Design review of the part built by this model. Coordinates are the model's own, in mm. A direction names the side the tool comes from. Coordinates: 2 decimals unless noted, no trailing zeros. Write each loop counter-clockwise with the first axis right and the second up, starting at its lowest first coordinate (ties: lowest second). Pieces come first, ordered by that corner, then holes. Notation, with made-up numbers: (12, 41) - (28, 41) arc R24 ccw to (28, 76) - close; hole circle Ø11 at (5, -30.5). An arc over 180 degrees is marked (long way). Use a Markdown table: item, result.
from build123d import *

# Parameters (mm, degrees)
BOSS_EXTRUDE1_DEPTH     = 20
CUT_EXTRUDE1_DEPTH      = 31.882754065
CUT_EXTRUDE1_DEPTH_BACK = 31.882754065
SKETCH2_R               = 2
SKETCH2_W               = 2
SKETCH2_H               = 5
FILLET1_R               = 2
FILLET2_R               = 0.5


with BuildPart() as part:
    # Sketch1 → Boss-Extrude1 (new body)
    with BuildSketch(Plane(origin=(0, 0, 0), x_dir=(1, 0, 0), z_dir=(0, 1, 0))):
        with BuildLine():
            Line((1.933321902, 6.18565004), (21.840134803, 7.875133355))
            ThreePointArc((21.840134803, 7.875133355), (22.103064319, 7.689578117), (21.96535024, 7.398721607))
            ThreePointArc((21.96535024, 7.398721607), (17.149860581, -0.069152491), (21.904969991, -7.575617618))
            ThreePointArc((21.904969991, -7.575617618), (22.040334019, -7.867575246), (21.775916667, -8.051004091))
            Line((21.775916667, -8.051004091), (1.883375697, -6.201039912))
            ThreePointArc((1.883375697, -6.201039912), (1.657998799, -5.979217339), (1.830264266, -5.714029464))
            ThreePointArc((1.830264266, -5.714029464), (5.999951224, -0.024193291), (1.876284769, 5.699083739))
            ThreePointArc((1.876284769, 5.699083739), (1.706163475, 5.965652202), (1.933321902, 6.18565004))
        make_face()
    extrude(amount=BOSS_EXTRUDE1_DEPTH)

    # Sketch2 → Cut-Extrude1 (cut, two sides: drawn at the far end of the back side and taken through both)
    with BuildSketch(Plane.XY.offset(-CUT_EXTRUDE1_DEPTH_BACK)):
        with Locations((14.149793513, 10)):
            Circle(SKETCH2_R)
        with Locations((10, 15)):
            Rectangle(SKETCH2_W, SKETCH2_H)
        with Locations((10, 5)):
            Rectangle(SKETCH2_W, SKETCH2_H)
    extrude(amount=CUT_EXTRUDE1_DEPTH + CUT_EXTRUDE1_DEPTH_BACK, mode=Mode.SUBTRACT)

    # Fillet1
    fillet1_edges = [part.edges().sort_by_distance(p)[0] for p in [
        (9, 5, 6.862870899),
        (9, 15, 6.862870899),
        (9, 15, -6.785396207),
        (9, 5, -6.785396207),
    ]]
    fillet(fillet1_edges, radius=FILLET1_R)

    # Fillet2
    fillet2_edges = [part.edges().sort_by_distance(p)[0] for p in [
        (11, 5, 7.048866663),
        (11, 15, 7.048866663),
        (11, 15, -6.955135414),
        (11, 5, -6.955135414),
    ]]
    fillet(fillet2_edges, radius=FILLET2_R)


solid = part.part
(1) Take a section at C-C on y = 10. Write out the cut boundary in (x, z), and give its area (3 significant figures).
Determined:
| item | result |
|---|---|
| outline | (1.83, 5.71) arc R6 cw to (1.88, -5.7) arc R0.25 ccw to (1.93, -6.19) - (12.15, -7.05) - (12.15, 7.16) - (1.88, 6.2) arc R0.25 ccw to start; (16.15, -7.39) - (21.84, -7.88) arc R0.25 ccw to (21.97, -7.4) arc R8.25 cw to (21.9, 7.58) arc R0.25 ccw to (21.78, 8.05) - (16.15, 7.53) - close |
| area | 140 mm2 |
(2) For pin 1 (5 mm diameter, centred on x = 4.5, y = 4, fed in from +Z); pin 2 (4 mm diameter, centred on x = 11.5, z = 4.5, fed in from -Y); pin 3 (5.5 mm diameter, centred on y = 16, z = -1.5, fed in from +X); pin 4 (8 mm diameter, centred on x = 7.5, y = 5.5, fed in from +Z), all flat-tipped, find the tip position at first contact; note any pin that passes through.
Determined:
| item | result |
|---|---|
| pin 1 | z = 6.67 |
| pin 2 | y = 0 |
| pin 3 | x = 18.39 |
| pin 4 | z = 7.1 |
(3) Draft analysis for pull direction Z (two halves, no side actions). For faces 1 (the flat face through (11, 5, 0)), 2 (the cylindrical face through (17.15, 9.86, -0.06)), 3 (the flat face through (11.97, 9.86, 7.14)), 4 (the cylindrical face through (8.336, 15.035, -6.097)), state which applies: +Z half, -Z half, draft (parallel to the pull), parting line (faces both ways), or undercut.
Determined:
| item | result |
|---|---|
| face 1 | draft |
| face 2 | undercut |
| face 3 | +Z half |
| face 4 | -Z half |
(4) Take a section at D-D on x = 14.25. Write out the cut boundary in (y, z).
Determined:
| item | result |
|---|---|
| outline | (0, -7.23) - (8, -7.23) - (8, 7.35) - (0, 7.35) - close; (12, -7.23) - (20, -7.23) - (20, 7.35) - (12, 7.35) - close |
(5) Machinability: for faces 5 (the flat face through (9, 5, 0)), 6 (the cylindrical face through (8.364, 4.965, 6.131)), 7 (the cylindrical face through (8.336, 5.035, -6.097)), 8 (the cylindrical face through (6, 10, 0)), 9 (the flat face through (12, 20, 0)), which of the approach directions +Z, -Z, +X, -X, +Y, -Y give a long, thin tool a straight path to every point of the face, cutting with its end or side? Answer none if there is none.
Determined:
| item | result |
|---|---|
| face 5 | +Z, -Z |
| face 6 | +Z |
| face 7 | -Z |
| face 8 | -X, +Y, -Y |
| face 9 | +Z, -Z, +X, -X, +Y |
(6) Take a section at A-A on x = 10.5. Write out the cut boundary in (y, z), and give its area (3 significant figures).
Determined:
| item | result |
|---|---|
| outline | (0, -6.91) - (2.5, -6.91) - (2.5, 7) - (0, 7) - close; (7.5, -6.91) - (12.5, -6.91) - (12.5, 7) - (7.5, 7) - close; (17.5, -6.91) - (20, -6.91) - (20, 7) - (17.5, 7) - close |
| area | 139 mm2 |
(7) For L1, parallel to Y at x = 9.75, z = -5; L2, parallel to Z at x = 11.5, y = 10.25; L3, parallel to X at y = 15.5, z = 3, list the stretches that pass through material, from the lowest coordinate up. Write a range as from..to.
Determined:
| item | result |
|---|---|
| L1 | 0..2.5, 7.5..12.5, 17.5..20 |
| L2 | -7..7.1 |
| L3 | 5.2..9, 11..17.68 |
(8) Take a section at B-B on z = -2.75. Write out the cut boundary in (x, y), and give its area (3 significant figures).
Determined:
| item | result |
|---|---|
| outline | (5.33, 0) - (17.66, 0) - (17.66, 20) - (5.33, 20) - close; hole (9, 2.5) - (11, 2.5) - (11, 7.5) - (9, 7.5) - close; hole (9, 12.5) - (11, 12.5) - (11, 17.5) - (9, 17.5) - close; hole circle Ø4 at (14.15, 10) |
| area | 214 mm2 |
